```python
from build123d import *

# Parameters (mm, degrees)
SKETCH_1_R          = 1.75
EXTRUDE_1_DEPTH     = 7.5
SKETCH_2_R          = 3
EXTRUDE_2_DEPTH     = 7.5
SKETCH_3_R          = 4.65
EXTRUDE_3_DEPTH     = 21.7
FILLET_1_R          = 1
EXTRUDE_4_DEPTH     = 3
CUT_EXTRUDE_START   = -2
SKETCH_5_R          = 4.65
SKETCH_5_R_2        = 2.75
CUT_EXTRUDE_1_DEPTH = 2
CHAMFER_1_SIZE      = 2


with BuildPart() as part:
    # 草图1 → 凸台-拉伸1 (new body)
    with BuildSketch(Plane(origin=(0, 0, 0), x_dir=(1, 0, 0), z_dir=(0, 1, 0))):
        with Locations(Location((0, 0, 0), (0, 0, 270))):
            Circle(SKETCH_1_R)
    extrude(amount=EXTRUDE_1_DEPTH)

    # 草图2 → 凸台-拉伸2 (add)
    with BuildSketch(Plane(origin=(0, 7.5, 0), x_dir=(1, 0, 0), z_dir=(0, 1, 0))):
        with Locations(Location((0, 0, 0), (0, 0, 270))):
            Circle(SKETCH_2_R)
    extrude(amount=EXTRUDE_2_DEPTH)

    # 草图3 → 凸台-拉伸3 (add)
    with BuildSketch(Plane(origin=(0, 15, 0), x_dir=(1, 0, 0), z_dir=(0, 1, 0))):
        with Locations(Location((0, 0, 0), (0, 0, 270))):
            Circle(SKETCH_3_R)
    extrude(amount=EXTRUDE_3_DEPTH)

    # 圆角1
    fillet_1_edges = [part.edges().sort_by_distance(p)[0] for p in [
        (0, 0, -1.75),
    ]]
    fillet(fillet_1_edges, radius=FILLET_1_R)

    # 草图4 → 凸台-拉伸4 (add)
    with BuildSketch(Plane.XZ.offset(-7.5)):
        Polygon((0, 4.618802154), (-4, 2.309401077), (-4, -2.309401077), (0, -4.618802154), (4, -2.309401077), (4, 2.309401077), align=None)
    extrude(amount=-EXTRUDE_4_DEPTH)

    # 草图5 → 切除-拉伸1 (cut)
    with BuildSketch(Plane(origin=(0, 36.7, 0), x_dir=(1, 0, 0), z_dir=(0, 1, 0)).offset(CUT_EXTRUDE_START)):
        with Locations(Location((0, 0, 0), (0, 0, 270))):
            Circle(SKETCH_5_R)
        with Locations(Location((0, 0, 0), (0, 0, 270))):
            Circle(SKETCH_5_R_2, mode=Mode.SUBTRACT)
    extrude(amount=CUT_EXTRUDE_1_DEPTH, mode=Mode.SUBTRACT)

    # 倒角1
    # the kernel refuses this chamfer: 2 mm, written as the material it takes off along each edge
    with BuildSketch(Plane(origin=(0, 15, 0), x_dir=(0, 0, 1), z_dir=(-1, 0, 0))) as chamfer_1_piece_1_section:
        Polygon((4.65 - CHAMFER_1_SIZE, 0), (4.65, CHAMFER_1_SIZE), (4.65, 0), align=None)
    chamfer_1_piece_1 = revolve(axis=Axis((0, 15, 0), (0, 1, 0)), mode=Mode.PRIVATE)
    chamfer_1_piece_1 = chamfer_1_piece_1 - Plane(origin=(0, 16.176636647, 0), x_dir=(0, 0, 1), z_dir=(0, -1, 0)) * Cylinder(3, 19, mode=Mode.PRIVATE)
    add(chamfer_1_piece_1, mode=Mode.SUBTRACT)


solid = part.part
```
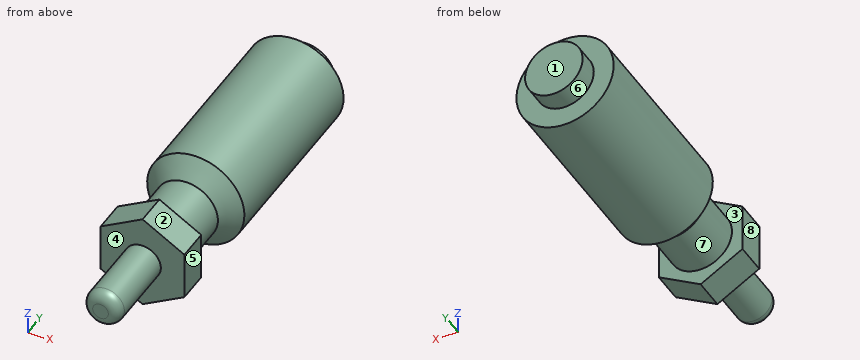
Can you work these out from the model? Positions are in its coordinate system, mm. Face numbers are marked on the shaded views. A direction names the side the tool comes from. Coordinates: 2 decimals unless noted, no trailing zeros. Loops run counter-clockwise (first coordinate to the right, second up) from the corner with the lowest first, then second, coordinate; pieces in that order, holes last.
Item 1: Suppose I cut it at A-A (y = 19.5). Please give me the cut outline in (x, z).
Answers below:
outline: circle Ø9.3 at (0, 0)
Item 2: Suppose I cut it at C-C (y = 9). Please give me the cut outline in (x, z), then the cut area to 3 significant figures.
Answers below:
outline: (-4, -2.31) - (0, -4.62) - (4, -2.31) - (4, 2.31) - (0, 4.62) - (-4, 2.31) - close
area: 55.4 mm2
Item 3: Please list where these lines run through material, in increasing order: L1, parallel to Y at x = -3.25, z = -0.75; L2, parallel to Y at x = 2.25, z = -3; L3, parallel to Z at x = 0.5, y = 33.
Answers below:
L1: y = 7.5 to 10.5, 15.69 to 34.7
L2: y = 7.5 to 10.5, 16.1 to 34.7
L3: z = -4.62 to 4.62
Item 4: Suppose I cut it at B-B (y = 5). Please give me the cut outline in (x, z), then the cut area to 3 significant figures.
Answers below:
outline: circle Ø3.5 at (0, 0)
area: 9.62 mm2
Item 5: If we mould it in two halves opening along Y, with no side actions, what happens to the marked faces 1, 2 and 3? For each: released by +Y, released by -Y, zero draft, split by the parting line, or undercut.
Answers below:
face 1: released by +Y
face 2: zero draft
face 3: undercut
Item 6: I'm going to push flat-ended pins straight in: pin 1 (5 mm diameter, centred on x = 0.5, y = 24.5, fed in from +Z); pin 2 (1.5 mm diameter, centred on x = 0, y = 7, fed in from -Z); pin 3 (1.5 mm diameter, centred on y = 9, z = 1, fed in from +X); pin 4 (2.5 mm diameter, centred on x = 0, z = 2.5, fed in from -Y). Where does each tip first touch, or does it pass through?
Answers below:
pin 1: stops at z = 4.65
pin 2: stops at z = -4.62
pin 3: stops at x = 4
pin 4: stops at y = 0.13
Item 7: Which directions (+Z, -Z, +X, -X, +Y, -Y) give clear straight access to the entire face, cutting with the end or side of a thin tool? Please do the marked faces 4, 5, 6, 7 and 8.
Answers below:
face 4: -Y
face 5: +Z, -Z, +X, -Y
face 6: +Y
face 7: none
face 8: +Z, -Z, -X, -Y
